```python
from build123d import *

# Parameters (mm, degrees)
F0_W     = 5
F0_H     = 5
F1_DEPTH = 10
F2_R     = 5
F2_W     = 5
F2_H     = 5
F3_DEPTH = 11
F5_DEPTH = 7.5


with BuildPart() as f1:
    # F0 (on Top) → F1 (new body)
    with BuildSketch(Plane.XY):
        Rectangle(F0_W, F0_H)
    extrude(amount=F1_DEPTH)

    # F2 (on face) → F3 (join)
    with BuildSketch(Plane.XY.offset(10)):
        Circle(F2_R)
        Rectangle(F2_W, F2_H, mode=Mode.SUBTRACT)
        Rectangle(F2_W, F2_H)
    extrude(amount=F3_DEPTH)

    # F4 (on face) → F5 (cut)
    with BuildSketch(Plane.XY.offset(21)):
        Polygon((1, 2.5), (-1, 2.5), (-1, 1), (-2.5, 1), (-2.5, -1), (-1, -1), (-1, -2.5), (1, -2.5), (1, -1), (2.5, -1), (2.5, 1), (1, 1), align=None)
    extrude(amount=-F5_DEPTH, mode=Mode.SUBTRACT)


solid = f1.part
```
Verification items for the finished model (mm, model axes). A direction names the side the tool comes from. Coordinates: 2 decimals unless noted, no trailing zeros. Order: outer loops, then holes, each group sorted by start corner. A loop starts at its lowest first (then second) coordinate and runs counter-clockwise, first axis right, second up. Notation, with made-up numbers: (-9, 74.25) -> (24, 74.25) arc R33 ccw to (24, 106.25) -> close; hole circle Ø3 at (12, 45). An arc over 180 degrees is marked (long way). Answer as CSV lines item,"result". Start each with the question number.
1) Cross-section at A-A, the plane z = 15. Record the boundary of the cut face in (x, y).
2) Release check for a two-part mould opening along Y. For faces 5 (the face through (1, 2, 17)), 6 (the face through (3, 0, 10)), 7 (the face through (0, 2.5, 5)) record: released by +Y, released by -Y, zero draft, split by the parting line, or undercut.
3) Cross-section at D-D, the plane z = 2.25. Record the boundary of the cut face in (x, y), then the cut area to 3 significant figures.
4) Material ranges on L1, parallel to Y at x = -0.5, z = 1.5; L2, parallel to Z at x = -3.5, y = 0; L3, parallel to Z at x = 0.5, y = 1.5, recorded low to high. Write a range as [from, to].
5) Cross-section at B-B, the plane x = 0. Record the boundary of the cut face in (y, z).
6) Set-up check for faces 1 (the face through (-2.5, 0, 17)), 2 (the face through (-2.5, 0, 5)), 3 (the face through (0, -2.5, 5)), 4 (the face through (2.5, 0, 5)): record each of +Z, -Z, +X, -X, +Y, -Y from which the full face is reachable in a straight line by a thin tool's end or side.
7) Gauge pin test, flat ends, axial feed: pin 1 Ø3 at (y, z) = (2, 15) entering from -X; pin 2 Ø5 at (y, z) = (-4, 17.5) entering from +X; pin 3 Ø0.8 at (y, z) = (2, 18) entering from -X. Record the tip position at first contact, or that the pin passes through.
Conclusion:
1,outline,"circle Ø10 at (0, 0); hole (-2.5, -1) -> (-1, -1) -> (-1, -2.5) -> (1, -2.5) -> (1, -1) -> (2.5, -1) -> (2.5, 1) -> (1, 1) -> (1, 2.5) -> (-1, 2.5) -> (-1, 1) -> (-2.5, 1) -> close"
2,face 5,"undercut"
2,face 6,"zero draft"
2,face 7,"released by +Y"
3,outline,"(-2.5, -2.5) -> (2.5, -2.5) -> (2.5, 2.5) -> (-2.5, 2.5) -> close"
3,area,"25.0 mm²"
4,L1,"y = [-2.5, 2.5]"
4,L2,"z = [10, 21]"
4,L3,"z = [0, 13.5]"
5,outline,"(-5, 10) -> (-2.5, 10) -> (-2.5, 0) -> (2.5, 0) -> (2.5, 10) -> (5, 10) -> (5, 21) -> (2.5, 21) -> (2.5, 13.5) -> (-2.5, 13.5) -> (-2.5, 21) -> (-5, 21) -> close"
6,face 1,"+Z"
6,face 2,"-Z, -X, +Y, -Y"
6,face 3,"-Z, +X, -X, -Y"
6,face 4,"-Z, +X, +Y, -Y"
7,pin 1,"stops at x = -4.97"
7,pin 2,"stops at x = 4.77"
7,pin 3,"stops at x = -4.74"
